The model under review builds one solid part; all positions refer to its coordinate system, in mm. A direction names the side the tool comes from. Coordinates: 2 decimals unless noted, no trailing zeros. Order: outer loops, then holes, each group sorted by start corner. A loop starts at its lowest first (then second) coordinate and runs counter-clockwise, first axis right, second up. Notation, with made-up numbers: (35.5, 51) -> (55.5, 51) arc R10 cw to (55.5, 64) -> close; hole circle Ø2 at (-17, -12). An arc over 180 degrees is marked (long way). Use one line per item in the form item = value.
Autodesk Inventor part; units mm, degrees
ref_plane "YZ Plane" through (0, 0, 0) normal (1, 0, 0) x (0, 1, 0)
ref_plane "XZ Plane" through (0, 0, 0) normal (0, 1, 0) x (-1, 0, 0)
ref_plane "XY Plane" through (0, 0, 0) normal (0, 0, 1) x (1, 0, 0)
sketch "Sketch1" plane through (0, 0, 0) normal (0, 0, 1) x (1, 0, 0)
  line L0 (57.15, 12.7) -> (-57.15, 12.7)
  line L1 (-57.15, 12.7) -> (-57.15, -12.7)
  line L2 (-57.15, -12.7) -> (57.15, -12.7)
  line L3 (57.15, -12.7) -> (57.15, 12.7)
  point P0 (0, 0)
  dimension "d0" = 114.3
  dimension "d1" = 25.4
extrude "Extrusion1" add sketch "Sketch1" against normal blind 3.175
sketch "Sketch2" plane through (-57.15, -12.7, 0) normal (-1, 0, 0) x (0, 0, 1)
  line L0 (0, 25.4) -> (0, 0)
  line L1 (0, 25.4) -> (-3.175, 25.4)
  line L2 (-3.175, 0) -> (-3.175, 25.4)
  line L3 (0, 0) -> (-3.175, 0)
  point P0 (0, 12.7)
sketch "Sketch3" plane through (0, 0, 0) normal (0, 0, 1) x (1, 0, 0)
  line L0 (57.15, -12.7) -> (-57.15, -12.7)
  line L1 (-57.15, 12.7) -> (-53.975, 12.7)
  line L2 (-53.975, 12.7) -> (-53.975, -12.7)
  line L3 (-53.975, -12.7) -> (-57.15, -12.7)
  line L4 (-57.15, -12.7) -> (-57.15, 12.7)
  point P0 (0, 0)
  dimension "d4" = 3.175
extrude "Extrusion2" cut sketch "Sketch2" against normal blind 3.175
extrude "Extrusion3" add sketch "Sketch3" against normal blind 76.2
sketch "Sketch4" plane through (0, 0, 0) normal (0, 0, 1) x (1, 0, 0)
  point P0 (0, 0)
sketch "Sketch5" plane through (0, 0, 0) normal (0, 0, 1) x (1, 0, 0)
  point P0 (0, 0)
sketch "Sketch6" plane through (57.15, -12.7, 0) normal (1, 0, 0) x (0, 0, -1)
  line L0 (0, 0) -> (0, 25.4)
  line L1 (0, 0) -> (3.175, 0)
  line L2 (3.175, 25.4) -> (3.175, 0)
  line L3 (0, 25.4) -> (3.175, 25.4)
  point P0 (0, 12.7)
extrude "Extrusion4" add sketch "Sketch6" along normal blind 12.7
sketch "Sketch7" plane through (0, 0, 0) normal (0, 0, 1) x (1, 0, 0)
  point P0 (0, 0)
sketch "Sketch8" plane through (0, 0, 0) normal (0, 0, 1) x (1, 0, 0)
  circle A0 centre (4.7498, 0) radius 3.2639
  point P0 (0, 0)
  dimension "d11" = 6.5278
extrude "Extrusion5" cut sketch "Sketch8" against normal blind 3.175
sketch "Sketch9" plane through (0, 0, 0) normal (0, 0, 1) x (1, 0, 0)
  circle A0 centre (30.1498, 0) radius 3.2639
  point P0 (0, 0)
  dimension "d14" = 6.5278
extrude "Extrusion6" cut sketch "Sketch9" against normal blind 3.175
sketch "Sketch10" plane through (0, 0, 0) normal (0, 0, 1) x (1, 0, 0)
  circle A0 centre (17.4498, 6.9088) radius 3.2639
  circle A1 centre (17.4498, -6.9088) radius 3.2639
  point P0 (0, 0)
  dimension "d17" = 6.5278
  dimension "d18" = 6.5278
extrude "Extrusion7" cut sketch "Sketch10" against normal blind 3.175
properties part number "lBracketForLiftingBar"
Item 1: To check wall thickness, follow L1, parallel to Z at x = -45.5, y = 7.75 (3 decimals); L2, parallel to X at y = -3.5, z = -6 (3 decimals). State the ranges of each line that lie inside material, in increasing order. Write a range as from..to.
Results found:
L1 = -3.175..0
L2 = -57.15..-53.975
Item 2: We need section B-B (x = 6). Write out the cut boundary in (y, z) (3 decimals).
Results found:
outline = (-12.7, -3.175) -> (-3.015, -3.175) -> (-3.015, 0) -> (-12.7, 0) -> close; (3.015, -3.175) -> (12.7, -3.175) -> (12.7, 0) -> (3.015, 0) -> close
Item 3: Clearance check with flat-ended pins moving along their axes: pin 1 (12.5 mm diameter, centred on x = 30, y = 4.5, fed in from -Z) (3 decimals); pin 2 (4 mm diameter, centred on y = -8, z = -31.5, fed in from +X) (3 decimals). State where each tip first meets the part, or that it passes through.
Results found:
pin_1 = -3.175
pin_2 = -53.975
Item 4: Draft analysis for pull direction Y (two halves, no side actions). For faces 1 (the face through (20.465, -8.159, -1.565)), 2 (the face through (-22, -12.7, -1)), 3 (the face through (-57.15, 0, -38)), 4 (the face through (20.563, 7.889, -1.565)), state which applies: released by +Y, released by -Y, zero draft, split by the parting line, or undercut.
Results found:
face_1 = undercut
face_2 = released by -Y
face_3 = zero draft
face_4 = undercut
Item 5: Tool access review of faces 5 (the face through (7, -3, -3.175)), 6 (the face through (7.765, -1.25, -1.565)): name each direction out of +Z, -Z, +X, -X, +Y, -Y from which nothing blocks a thin tool from reaching the whole face with its end or side.
Results found:
face_5 = -Z, +X, +Y, -Y
face_6 = +Z, -Z
Item 6: We need section D-D (z = -4.5). Write out the cut boundary in (x, y) (3 decimals), plus the area to 3 significant figures.
Results found:
outline = (-57.15, -12.7) -> (-53.975, -12.7) -> (-53.975, 12.7) -> (-57.15, 12.7) -> close
area = 80.6 mm²
Item 7: We need section A-A (y = 0). Write out the cut boundary in (x, z) (3 decimals).
Results found:
outline = (-57.15, -76.2) -> (-53.975, -76.2) -> (-53.975, -3.175) -> (1.486, -3.175) -> (1.486, 0) -> (-57.15, 0) -> close; (8.014, -3.175) -> (26.886, -3.175) -> (26.886, 0) -> (8.014, 0) -> close; (33.414, -3.175) -> (69.85, -3.175) -> (69.85, 0) -> (33.414, 0) -> close
Item 8: We need section C-C (x = -30.5). Write out the cut boundary in (y, z) (3 decimals).
Results found:
outline = (-12.7, -3.175) -> (12.7, -3.175) -> (12.7, 0) -> (-12.7, 0) -> close
